Print and shaded views of the part. All mm, measured from the part's lowest x, y and z. A direction names the side the tool comes from. Round coordinates to 2 decimals unless told otherwise and drop trailing zeros. Loops run counter-clockwise (first coordinate to the right, second up) from the corner with the lowest first, then second, coordinate; pieces in that order, holes last. Notation, with made-up numbers: M 10,80 L 66,80 A32 ccw 66,113 Z; hole C 10,-22 d9. An arc over 180 degrees is marked long. One line per item, written item: value. Start each with the question number.
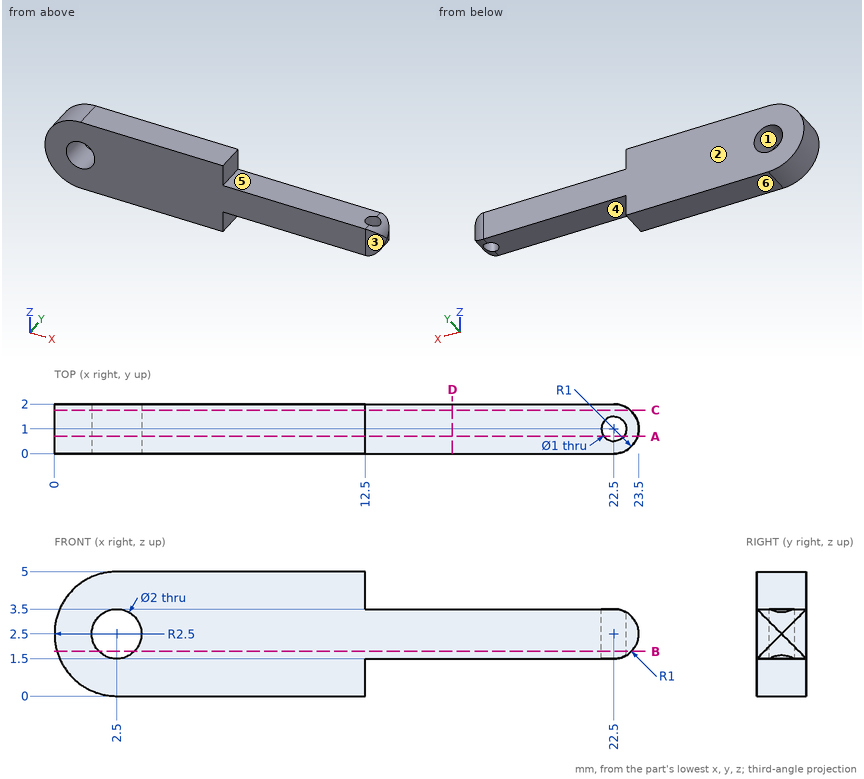
(1) Slice it at A-A, the plane y = 0.7. List the corners of the cut face in (x, z).
(2) Probe L1, parallel to X at y = 1, z = 2.4; L2, parallel to X at y = 1.4, z = 1.65; L3, parallel to Y at x = 22.5, z = 2.9. List the from-to ranges inside material, lowest first.
(3) Slice it at C-C, the plane y = 1.75. List the corners of the cut face in (x, z), and give its area (3 significant figures).
(4) Flat gauge pins, fed straight in: P1, Ø1.8, axis at x = 2.5, z = 2.5, coming from the -Y side; P2, Ø1, axis at x = 18.5, y = 1, coming from the +Z side; P3, Ø0.8, axis at y = 1, z = 0.5, coming from the +X side. Where does each tip first touch, or does it go through?
(5) Which spindle directions (+Z, -Z, +X, -X, +Y, -Y) get a long thin tool onto all of the face, cutting with end or side? Do the marked faces 4, 5 and 6. Say none if no direction does.
(6) Slice it at B-B, the plane z = 1.8. List the corners of the cut face in (x, y).
(7) Slice it at D-D, the plane x = 16. List the corners of the cut face in (y, z), and give its area (3 significant figures).
(8) Mould opens along X. For the marked faces 1, 2 and 3 say: pulls with the +X half, pulls with the -X half, needs draft (parallel to the pull), parting line crosses it, or undercut.
Check result:
1. outline: M 2.5,0 L 12.5,0 L 12.5,1.5 L 22.1,1.5 L 22.1,3.5 L 12.5,3.5 L 12.5,5 L 2.5,5 A2.5 ccw Z; M 22.9,1.58 A1 ccw 23.45,2.2 L 23.45,2.8 A1 ccw 22.9,3.42 Z; hole C 2.5,2.5 d2
2. L1: x = 0 to 1.51, 3.49 to 22, 23 to 23.49
2. L2: x = 0.15 to 1.97, 3.03 to 22.2, 22.8 to 23.03
2. L3: y = 0 to 0.5, 1.5 to 2
3. outline: M 2.5,0 L 12.5,0 L 12.5,1.5 L 22.5,1.5 A1 ccw 23.16,1.75 L 23.16,3.25 A1 ccw 22.5,3.5 L 12.5,3.5 L 12.5,5 L 2.5,5 A2.5 ccw Z; hole C 2.5,2.5 d2
3. area: 77.9 mm^2
4. P1: passes through
4. P2: stops at z = 3.5
4. P3: stops at x = 12.5
5. face 4: -Z, +X, +Y, -Y
5. face 5: +Z, +X, +Y, -Y
5. face 6: -Z, +X, -X, +Y, -Y
6. outline: M 0.1,0 L 1.79,0 L 1.79,2 L 0.1,2 Z; M 3.21,0 L 22.5,0 A1 ccw 23.21,0.3 L 23.21,1.7 A1 ccw 22.5,2 L 3.21,2 Z; hole C 22.5,1 d1
7. outline: M 0,1.5 L 2,1.5 L 2,3.5 L 0,3.5 Z
7. area: 4.00 mm^2
8. face 1: undercut
8. face 2: needs draft
8. face 3: pulls with the +X half
